```python
from build123d import *

# Parameters (mm, degrees)
SKETCH1_R           = 3.15
SKETCH1_R_2         = 8.25
BOSS_EXTRUDE1_DEPTH = 2
BOSS_EXTRUDE2_DEPTH = 45
SKETCH3_R           = 8.25
CUT_EXTRUDE1_DEPTH  = 104.812694214
SKETCH4_W           = 30
SKETCH4_H           = 7.560001502
BOSS_EXTRUDE3_DEPTH = 30
SKETCH5_R           = 1.945
CUT_EXTRUDE2_DEPTH  = 130.889649736
CUT_EXTRUDE3_DEPTH  = 120.90444312
SKETCH10_W          = 23
SKETCH10_H          = 46
BOSS_EXTRUDE4_DEPTH = 21.2
SKETCH11_W          = 22.207892016
SKETCH11_H          = 46.715728752
CUT_EXTRUDE4_DEPTH  = 119.384613888
SKETCH12_W          = 0.6
SKETCH12_H          = 23.8
CUT_EXTRUDE5_DEPTH  = 118.813722566
BOSS_EXTRUDE5_DEPTH = 42
SKETCH14_R          = 14
CUT_EXTRUDE6_DEPTH  = 119.420577709
SKETCH15_R          = 2
CUT_EXTRUDE7_DEPTH  = 119.420577709


with BuildPart() as part:
    # Sketch1 → Boss-Extrude1 (new body)
    with BuildSketch(Plane(origin=(0, 0, 0), x_dir=(1, 0, 0), z_dir=(0, 1, 0))):
        Polygon((-48.732366868, 38.443096859), (21.267633132, 38.443096859), (21.267633132, -31.556903141), (21.267633132, -79.857572586), (-48.732366868, -79.857572586), (-48.732366868, -31.556903141), align=None)
        with Locations(Location((-42.016638116, 31.727368106, 0), (0, 0, 270))):
            Circle(SKETCH1_R, mode=Mode.SUBTRACT)
        with Locations(Location((14.551904379, 31.727368106, 0), (0, 0, 270))):
            Circle(SKETCH1_R, mode=Mode.SUBTRACT)
        with Locations(Location((14.551904379, -24.841174389, 0), (0, 0, 270))):
            Circle(SKETCH1_R, mode=Mode.SUBTRACT)
        with Locations(Location((-42.016638116, -24.841174389, 0), (0, 0, 270))):
            Circle(SKETCH1_R, mode=Mode.SUBTRACT)
        with Locations(Location((-13.732366868, -19.556903141, 0), (0, 0, 270))):
            Circle(SKETCH1_R_2, mode=Mode.SUBTRACT)
    extrude(amount=BOSS_EXTRUDE1_DEPTH)

    # Sketch2 → Boss-Extrude2 (add)
    with BuildSketch(Plane(origin=(0, 2, 0), x_dir=(1, 0, 0), z_dir=(0, 1, 0))):
        Polygon((-28.732366868, 20.263098361), (1.267633132, 20.263098361), (1.267633132, 8.916503275), (-3.732366868, 8.916503275), (-3.732366868, -31.556903141), (-22.732366868, -31.556903141), (-22.732366868, 5.987652995), (-22.732366868, 8.916503275), (-28.732366868, 8.916503275), (-28.732366868, 9.103096859), align=None)
    extrude(amount=BOSS_EXTRUDE2_DEPTH)

    # Sketch3 → Cut-Extrude1 (cut, through all)
    with BuildSketch(Plane.XZ.offset(-2)):
        with Locations(Location((-13.732366868, 19.556903141, 0), (0, 0, 270))):
            Circle(SKETCH3_R)
    extrude(amount=-CUT_EXTRUDE1_DEPTH, mode=Mode.SUBTRACT)

    # Sketch4 → Boss-Extrude3 (add)
    with BuildSketch(Plane(origin=(0, 47, 0), x_dir=(1, 0, 0), z_dir=(0, 1, 0))):
        with Locations((-13.732366868, 16.48309761)):
            Rectangle(SKETCH4_W, SKETCH4_H)
    extrude(amount=BOSS_EXTRUDE3_DEPTH)

    # Sketch5 → Cut-Extrude2 (cut, through all)
    with BuildSketch(Plane.XY.offset(-12.703096859)):
        with Locations((-22.527366868, 54.069519899)):
            Circle(SKETCH5_R)
        with Locations((-6.937366868, 54.069519899)):
            Circle(SKETCH5_R)
    extrude(amount=-CUT_EXTRUDE2_DEPTH, mode=Mode.SUBTRACT)

    # Sketch6 → Cut-Extrude3 (cut, through all)
    with BuildSketch(Plane(origin=(0, 2, 0), x_dir=(1, 0, 0), z_dir=(0, 1, 0))):
        Polygon((-48.732366868, -18.841174389), (-22.732366868, -18.841174389), (-22.732366868, 8.916503275), (-28.732366868, 8.916503275), (-28.732366868, 12.703096859), (-28.732366868, 20.263098361), (1.267633132, 20.263098361), (1.267633132, 8.916503275), (-3.732366868, 8.916503275), (-3.732366868, -18.841174389), (21.267633132, -18.841174389), (21.267633132, 38.443096859), (-48.732366868, 38.443096859), align=None)
        Polygon((-48.732366868, -30.841174389), (-44.940258884, -30.841174389), (-44.940258884, -77.556903141), (0.267633132, -77.556903141), (0.267633132, -30.841174389), (21.267633132, -30.841174389), (21.267633132, -79.857572586), (-48.732366868, -79.857572586), align=None)
    extrude(amount=-CUT_EXTRUDE3_DEPTH, mode=Mode.SUBTRACT)

    # Sketch10 → Boss-Extrude4 (add)
    with BuildSketch(Plane(origin=(0, 2, 0), x_dir=(1, 0, 0), z_dir=(0, 1, 0))):
        with Locations((-11.232366868, -54.556903141)):
            Rectangle(SKETCH10_W, SKETCH10_H)
    extrude(amount=BOSS_EXTRUDE4_DEPTH)

    # Sketch11 → Cut-Extrude4 (cut, through all)
    with BuildSketch(Plane(origin=(0, 2, 0), x_dir=(1, 0, 0), z_dir=(0, 1, 0))):
        with Locations((-33.836312876, -54.199038765)):
            Rectangle(SKETCH11_W, SKETCH11_H)
    extrude(amount=-CUT_EXTRUDE4_DEPTH, mode=Mode.SUBTRACT)

    # Sketch12 → Cut-Extrude5 (cut, through all)
    with BuildSketch(Plane.ZY.offset(22.732366868)):
        with Locations((31.256903141, 35.1)):
            Rectangle(SKETCH12_W, SKETCH12_H)
    extrude(amount=-CUT_EXTRUDE5_DEPTH, mode=Mode.SUBTRACT)

    # Sketch13 → Boss-Extrude5 (add)
    with BuildSketch(Plane(origin=(0, 23.2, 0), x_dir=(1, 0, 0), z_dir=(0, 1, 0))):
        Polygon((0.267633132, -77.556903141), (-22.732366868, -77.556903141), (-22.732366868, -74.156903141), (-3.132366868, -74.156903141), (-3.132366868, -33.22347783), (0.267633132, -33.22347783), (0.267633132, -74.156903141), align=None)
    extrude(amount=BOSS_EXTRUDE5_DEPTH)

    # Sketch14 → Cut-Extrude6 (cut, through all)
    with BuildSketch(Plane.ZY.offset(3.132366868)):
        with Locations((52.556903141, 44.785296811)):
            Circle(SKETCH14_R)
    extrude(amount=-CUT_EXTRUDE6_DEPTH, mode=Mode.SUBTRACT)

    # Sketch15 → Cut-Extrude7 (cut, through all)
    with BuildSketch(Plane.ZY.offset(3.132366868)):
        with Locations((68.056903141, 29.285296811)):
            Circle(SKETCH15_R)
        with Locations((37.056903141, 29.285296811)):
            Circle(SKETCH15_R)
        with Locations((37.056903141, 60.285296811)):
            Circle(SKETCH15_R)
        with Locations((68.056903141, 60.285296811)):
            Circle(SKETCH15_R)
    extrude(amount=-CUT_EXTRUDE7_DEPTH, mode=Mode.SUBTRACT)


solid = part.part
```
Here's how the part is built. I have some questions about the finished solid (model axes, mm). A direction names the side the tool comes from. Coordinates: 2 decimals unless noted, no trailing zeros. Write each loop counter-clockwise with the first axis right and the second up, starting at its lowest first coordinate (ties: lowest second). Pieces come first, ordered by that corner, then holes. Notation, with made-up numbers: (68.5, 35) - (105.5, 35) arc R12 ccw to (105.5, 44) - close; hole circle Ø7 at (34.25, 83.5). An arc over 180 degrees is marked (long way). One line per item, written item: value.
1) Suppose I cut it at C-C on z = 29.5. Write out the boundary of the cut face in (x, y), and give its area (3 significant figures).
Model answer:
outline: (-48.73, 0) - (21.27, 0) - (21.27, 2) - (-3.73, 2) - (-3.73, 47) - (-22.73, 47) - (-22.73, 2) - (-48.73, 2) - close
area: 995 mm²
2) We'd pull the mould along Y, two halves only. Please class faces 1 (the flat face through (9, 2, 25)), 2 (the cylindrical face through (-1.456, 29.886, 69.965)), 3 (the flat face through (0.268, 25, 55)), 4 (the cylindrical face through (-1.456, 28.519, 38.904)): pulls with the +Y half, pulls with the -Y half, needs draft (parallel to the pull), parting line crosses it, or undercut.
Model answer:
face 1: pulls with the +Y half
face 2: undercut
face 3: needs draft
face 4: undercut
3) Suppose I cut it at D-D on x = -44. Write out the boundary of the cut face in (y, z), and give its area (3 significant figures).
Model answer:
outline: (0, 18.84) - (2, 18.84) - (2, 22.39) - (0, 22.39) - close; (0, 27.29) - (2, 27.29) - (2, 30.84) - (0, 30.84) - close
area: 14.2 mm²
4) Suppose I cut it at B-B on y = 37.5. Write out the boundary of the cut face in (x, z), and give its area (3 significant figures).
Model answer:
outline: (-28.73, -20.26) - (1.27, -20.26) - (1.27, -8.92) - (-3.73, -8.92) - (-3.73, 30.96) - (-22.73, 30.96) - (-22.73, -8.92) - (-28.73, -8.92) - close; (-22.73, 74.16) - (-3.13, 74.16) - (-3.13, 64.51) - (0.27, 64.51) - (0.27, 77.56) - (-22.73, 77.56) - close; (-3.13, 33.22) - (0.27, 33.22) - (0.27, 40.6) - (-3.13, 40.6) - close; hole circle Ø16.5 at (-13.73, 19.56)
area: 1,020 mm²
5) Suppose I cut it at A-A on y = 25. Write out the boundary of the cut face in (x, z).
Model answer:
outline: (-28.73, -20.26) - (1.27, -20.26) - (1.27, -8.92) - (-3.73, -8.92) - (-3.73, 30.96) - (-22.73, 30.96) - (-22.73, -8.92) - (-28.73, -8.92) - close; (-22.73, 74.16) - (-3.13, 74.16) - (-3.13, 33.22) - (0.27, 33.22) - (0.27, 77.56) - (-22.73, 77.56) - close; hole circle Ø16.5 at (-13.73, 19.56)
6) I need wall thicknesses on line 1 along Z through (x, y) = (-3, 57); line 2 along Z through (x, y) = (-9, 24); line 3 along X through (y, z) = (36, 9). Which ranges of each line are inside material? Lowest first, please.
Model answer:
line 1: z = -20.26 to -12.7, 33.22 to 45.72, 59.4 to 77.56
line 2: z = -20.26 to 12.8, 26.31 to 30.96, 74.16 to 77.56
line 3: x = -22.73 to -3.73
7) I'm going to push flat-ended pins straight in: P1, Ø23.5, axis at y = 19.5, z = 47, coming from the +X side; P2, Ø1.6, axis at x = -38, y = 1.5, coming from the -Z side; P3, Ø3, axis at y = 47, z = 15, coming from the +X side; P4, Ø3.5, axis at x = -41.5, z = 24.5, coming from the +Y side. Where does each tip first touch, or does it pass through?
Model answer:
P1: stops at x = 0.27
P2: stops at z = 18.84
P3: stops at x = -3.73
P4: passes through
8) On a 3-axis mill with a long thin cutter (end or side, diameter ignored), from which of +Z, -Z, +X, -X, +Y, -Y can I reach the whole of each face in a straight line? I mean faces 5 (the flat face through (-13, 44, 74.157)), 6 (the flat face through (-2.7, 65.2, 60.2)), 7 (the cylindrical face through (-21.63, 52.344, -16.43)), 8 (the flat face through (-14, 62, -12.703)). Say none if no direction works.
Model answer:
face 5: -X, +Y
face 6: +Z, +X, -X, +Y
face 7: -Z
face 8: +X, -X, +Y
